Can you work these out from the model? Positions are in its coordinate system, mm. Face numbers are marked on the shaded views. A direction names the side the tool comes from. Coordinates: 2 decimals unless noted, no trailing zeros. Loops run counter-clockwise (first coordinate to the right, second up) from the corner with the lowest first, then second, coordinate; pieces in that order, holes last.
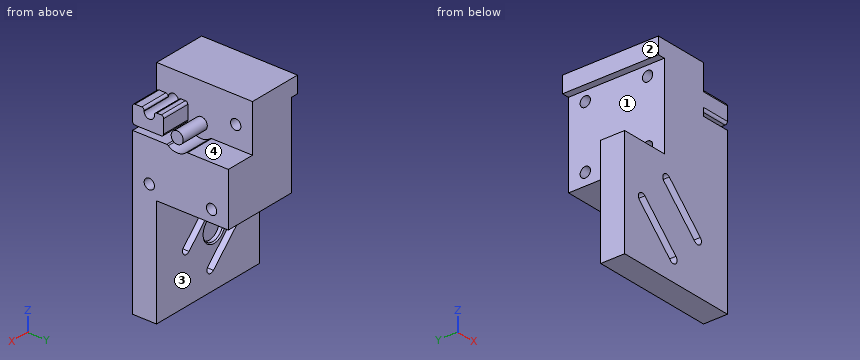
```python
from build123d import *

# Parameters (mm, degrees)
SKETCH3_W             = 13.49028586
SKETCH3_H             = 10
BOSS_EXTRUDE1_DEPTH   = 22
SKETCH3_W_2           = 3
BOSS_EXTRUDE1_2_DEPTH = 22
BOSS_EXTRUDE1_3_DEPTH = 22
SKETCH4_W             = 27.150730292
SKETCH4_H             = 10
BOSS_EXTRUDE2_DEPTH   = 3
SKETCH5_W             = 27.150730292
SKETCH5_H             = 10
BOSS_EXTRUDE3_DEPTH   = 3
SKETCH7_W             = 12.1
SKETCH7_H             = 14.76
BOSS_EXTRUDE4_DEPTH   = 10
BOSS_EXTRUDE5_DEPTH   = 10
SKETCH15_R            = 1.915111108
CUT_EXTRUDE4_DEPTH    = 320.517471197
SKETCH18_W            = 12.1
SKETCH18_H            = 14.76
BOSS_EXTRUDE6_DEPTH   = 30
M4_CLEARANCE_HOLE1_D  = 4.3
CUT_EXTRUDE7_DEPTH    = 5
SKETCH17_R            = 5
CUT_EXTRUDE6_DEPTH    = 2
CHAMFER1_SIZE         = 0.5
SKETCH24_W            = 5
SKETCH24_H            = 40
CUT_EXTRUDE8_DEPTH    = 12.1
SKETCH25_R            = 2.5
BOSS_EXTRUDE10_DEPTH  = 12.1
CUT_EXTRUDE10_START   = -12.1
SKETCH31_R            = 5.628705003
SKETCH31_R_2          = 2.5
CUT_EXTRUDE10_DEPTH   = 12.1
FILLET1_R             = 1


with BuildPart() as part:
    # Sketch3 → Boss-Extrude1 (new body)
    with BuildSketch(Plane(origin=(-188.9, 0, 188.9), x_dir=(0.7071067811865475, 0, 0.7071067811865477), z_dir=(-0.7071067811865477, 0, 0.7071067811865475))):
        with Locations((0, -11.606969024)):
            Rectangle(SKETCH3_W, SKETCH3_H)
    extrude(amount=-BOSS_EXTRUDE1_DEPTH)



with BuildPart() as body_2:
    # Sketch3 → Boss-Extrude1 2 (new body)
    with BuildSketch(Plane(origin=(-188.9, 0, 188.9), x_dir=(0.7071067811865475, 0, 0.7071067811865477), z_dir=(-0.7071067811865477, 0, 0.7071067811865475))):
        with Locations((12.075365146, -11.606969024)):
            Rectangle(SKETCH3_W_2, SKETCH3_H)
    extrude(amount=-BOSS_EXTRUDE1_2_DEPTH)


with BuildPart() as body_3:
    # Sketch3 → Boss-Extrude1 3 (new body)
    with BuildSketch(Plane(origin=(-188.9, 0, 188.9), x_dir=(0.7071067811865475, 0, 0.7071067811865477), z_dir=(-0.7071067811865477, 0, 0.7071067811865475))):
        with Locations((-12.075365146, -11.606969024)):
            Rectangle(SKETCH3_W_2, SKETCH3_H)
    extrude(amount=-BOSS_EXTRUDE1_3_DEPTH)


with BuildPart() as part_1:
    add(part.part)

    add(body_2.part)  # Boss-Extrude2 merges body 2

    add(body_3.part)  # Boss-Extrude2 merges body 3
    # Sketch4 → Boss-Extrude2 (add)
    with BuildSketch(Plane(origin=(-188.9, 0, 188.9), x_dir=(0.7071067811865472, 0, 0.7071067811865479), z_dir=(-0.7071067811865479, 0, 0.7071067811865472))):
        with Locations((0, -11.606969024)):
            Rectangle(SKETCH4_W, SKETCH4_H)
    extrude(amount=BOSS_EXTRUDE2_DEPTH)

    # Sketch5 → Boss-Extrude3 (add)
    with BuildSketch(Plane(origin=(-173.343650814, 0, 173.343650814), x_dir=(-0.7071067811865472, 0, -0.7071067811865479), z_dir=(0.7071067811865479, 0, -0.7071067811865472))):
        with Locations((0, -11.606969024)):
            Rectangle(SKETCH5_W, SKETCH5_H)
    extrude(amount=BOSS_EXTRUDE3_DEPTH)

    # Sketch7 → Boss-Extrude4 (add)
    with BuildSketch(Plane(origin=(0, -6.606969024, 0), x_dir=(1, 0, 0), z_dir=(0, 1, 0))):
        Polygon((-183.9, -239), (-186.9, -239), (-186.9, -245.88), (-147.25, -245.88), (-147.25, -161.623097719), (-180.821563222, -161.623097719), (-161.623097719, -180.821563222), (-181.422087592, -200.620553095), (-200.620553095, -181.422087592), (-200.620553095, -203.8), (-183.9, -203.8), align=None)
        with Locations((-158.3, -233.5)):
            Rectangle(SKETCH7_W, SKETCH7_H, mode=Mode.SUBTRACT)
    extrude(amount=-BOSS_EXTRUDE4_DEPTH)

    # Sketch13 → Boss-Extrude5 (add)
    with BuildSketch(Plane(origin=(0, -6.606969024, 0), x_dir=(1, 0, 0), z_dir=(0, 1, 0))):
        Polygon((-203.8, -203.8), (-200.620553095, -203.8), (-200.620553095, -181.422087592), (-180.821563222, -161.623097719), (-147.25, -161.623097719), (-147.25, -158.443650814), (-203.8, -158.443650814), align=None)
    extrude(amount=-BOSS_EXTRUDE5_DEPTH)

    # Sketch15 → Cut-Extrude4 (cut, through all)
    with BuildSketch(Plane(origin=(0, -6.606969024, 0), x_dir=(1, 0, 0), z_dir=(0, 1, 0))):
        with Locations((-179.467375171, -167.219926457)):
            Circle(SKETCH15_R)
        with Locations((-167.219926457, -179.467375171)):
            Circle(SKETCH15_R)
        with Locations((-195.023724357, -182.776275643)):
            Circle(SKETCH15_R)
        with Locations((-182.776275643, -195.023724357)):
            Circle(SKETCH15_R)
    extrude(amount=-CUT_EXTRUDE4_DEPTH, mode=Mode.SUBTRACT)

    # Sketch18 → Boss-Extrude6 (add)
    with BuildSketch(Plane(origin=(0, -6.606969024, 0), x_dir=(1, 0, 0), z_dir=(0, 1, 0))):
        Polygon((-183.9, -203.8), (-147.25, -203.8), (-147.25, -245.88), (-186.9, -245.88), (-186.9, -239), (-183.9, -239), align=None)
        with Locations((-158.3, -233.5)):
            Rectangle(SKETCH18_W, SKETCH18_H, mode=Mode.SUBTRACT)
    extrude(amount=BOSS_EXTRUDE6_DEPTH)

    # M4 Clearance Hole1 (through all)
    with Locations(Plane(origin=(-147.25, 0, 0), x_dir=(0, 0, -1), z_dir=(1, 0, 0))):
        with Locations((-234.9, 16.393030976), (-208.9, -9.606969024), (-234.9, -9.606969024), (-208.9, 16.393030976)):
            Hole(M4_CLEARANCE_HOLE1_D / 2)

    # Sketch22 → Cut-Extrude7 (cut)
    with BuildSketch(Plane(origin=(-147.25, 0, 0), x_dir=(0, 0, -1), z_dir=(1, 0, 0))):
        Polygon((-245.88, 23.393030976), (-245.88, -16.606969024), (-158.443650814, -16.606969024), (-158.443650814, -6.606969024), (-203.8, -6.606969024), (-203.8, 23.393030976), align=None)
    extrude(amount=-CUT_EXTRUDE7_DEPTH, mode=Mode.SUBTRACT)

    # Sketch17 → Cut-Extrude6 (cut)
    with BuildSketch(Plane(origin=(0, -6.606969024, 0), x_dir=(1, 0, 0), z_dir=(0, 1, 0))):
        with Locations(Location((-181.121825407, -181.121825407, 0), (0, 0, 270))):
            Circle(SKETCH17_R)
    extrude(amount=-CUT_EXTRUDE6_DEPTH, mode=Mode.SUBTRACT)

    # Chamfer1
    chamfer1_edges = [part_1.edges().sort_by_distance(p)[0] for p in [
        (-181.121825407, -6.606969024, 176.121825407),
    ]]
    chamfer(chamfer1_edges, length=CHAMFER1_SIZE)

    # Sketch24 → Cut-Extrude8 (cut)
    with BuildSketch(Plane(origin=(-152.25, 0, 0), x_dir=(0, 0, -1), z_dir=(1, 0, 0))):
        with Locations((-243.38, 3.393030976)):
            Rectangle(SKETCH24_W, SKETCH24_H)
    extrude(amount=-CUT_EXTRUDE8_DEPTH, mode=Mode.SUBTRACT)

    # Sketch25 → Boss-Extrude10 (add)
    with BuildSketch(Plane(origin=(-164.35, 0, 0), x_dir=(0, 0, -1), z_dir=(1, 0, 0))):
        with Locations(Location((-230.14, 2.021735979, 0), (0, 0, 270))):
            Circle(SKETCH25_R)
        with BuildLine():
            Line((-228.41, -3.606969024), (-236.12, -3.606969024))
            Line((-236.12, -3.606969024), (-236.12, -7.456969024))
            Line((-236.12, -7.456969024), (-234.9, -7.456969024))
            ThreePointArc((-234.9, -7.456969024), (-232.75, -9.606969024), (-234.9, -11.756969024))
            Line((-234.9, -11.756969024), (-236.12, -11.756969024))
            Line((-236.12, -11.756969024), (-236.12, -16.606969024))
            Line((-236.12, -16.606969024), (-228.41, -16.606969024))
            Line((-228.41, -16.606969024), (-228.41, -3.606969024))
        make_face()
    extrude(amount=BOSS_EXTRUDE10_DEPTH)

    # Sketch31 → Cut-Extrude10 (cut)
    with BuildSketch(Plane(origin=(-152.25, 0, 0), x_dir=(0, 0, -1), z_dir=(1, 0, 0)).offset(CUT_EXTRUDE10_START)):
        with Locations((-230.14, 2.021735979)):
            Circle(SKETCH31_R)
        with Locations(Location((-230.14, 2.021735979, 0), (0, 0, 270))):
            Circle(SKETCH31_R_2, mode=Mode.SUBTRACT)
    extrude(amount=CUT_EXTRUDE10_DEPTH, mode=Mode.SUBTRACT)

    # Fillet1
    fillet1_edges = [part_1.edges().sort_by_distance(p)[0] for p in [
        (-158.3, -16.606969024, 228.41),
        (-158.3, -3.606969024, 228.41),
        (-158.3, -3.606969024, 236.12),
        (-158.3, -7.456969024, 236.12),
        (-158.3, -11.756969024, 236.12),
        (-158.3, -16.606969024, 236.12),
        (-158.3, 5.961522777, 226.12),
        (-158.3, -1.918050819, 226.12),
    ]]
    fillet(fillet1_edges, radius=FILLET1_R)


solid = part_1.part
```
(1) I want a section at D-D on z = 195.5. Write out the boundary of the cut face in (x, y), then the cut area to 3 significant figures.
Check values:
outline: (-203.8, -16.61) - (-184.63, -16.61) - (-184.63, -6.61) - (-203.8, -6.61) - close; (-180.54, -16.61) - (-152.25, -16.61) - (-152.25, -6.61) - (-180.54, -6.61) - close
area: 475 mm2
(2) If I drill on probe 1 along Z at (x, y) = (-183.5, 14.5); probe 2 along Z at (x, y) = (-180, 18); probe 3 along X at (y, z) = (-11.5, 184), over which ranges is the centre line in solid material (lowest first)?
Check values:
probe 1: z = 203.8 to 207.88, 209.92 to 233.88, 235.92 to 245.88
probe 2: z = 203.8 to 207.47, 210.33 to 233.47, 236.33 to 245.88
probe 3: x = -203.8 to -196.5, -193.54 to -174.46, -169.04 to -152.25
(3) I'm going to push flat-ended pins straight in: pin 1 (2.5 mm diameter, centred on y = -9.61, z = 234.9, fed in from -X); pin 2 (15 mm diameter, centred on x = -167.5, y = 15, fed in from -Z); pin 3 (3 mm diameter, centred on x = -183.5, z = 179, fed in from +Y); pin 4 (2.5 mm diameter, centred on x = -156.5, y = -13.5, fed in from +Z). Where does each tip first touch, or does it pass through?
Check values:
pin 1: passes through
pin 2: stops at z = 203.8
pin 3: stops at y = -8.61
pin 4: stops at z = 236.12
(4) I want a section at A-A on z = 208.9. Write out the boundary of the cut face in (x, y), then the cut area to 3 significant figures.
Check values:
outline: (-183.9, -16.61) - (-152.25, -16.61) - (-152.25, -11.76) - (-183.9, -11.76) - close; (-183.9, -7.46) - (-152.25, -7.46) - (-152.25, 14.24) - (-183.9, 14.24) - close; (-183.9, 18.54) - (-152.25, 18.54) - (-152.25, 23.39) - (-183.9, 23.39) - close
area: 994 mm2
(5) Which directions (+Z, -Z, +X, -X, +Y, -Y) give clear straight access to the entire face, cutting with the end or side of a thin tool? Please do the marked faces 1, 2, 3 and 4.
Check values:
face 1: -X, +Y, -Y
face 2: +Z, -X, +Y, -Y
face 3: -Z, +X, -X, +Y
face 4: +Z, +X, +Y, -Y
(6) I want a section at C-C on y = 11. Write out the boundary of the cut face in (x, z), then the cut area to 3 significant figures.
Check values:
outline: (-186.9, 239) - (-183.9, 239) - (-183.9, 203.8) - (-152.25, 203.8) - (-152.25, 226.12) - (-164.35, 226.12) - (-164.35, 245.88) - (-186.9, 245.88) - close
area: 1,110 mm2
(7) I want a section at B-B on x = -174. Write out the boundary of the cut face in (y, z).
Check values:
outline: (-16.61, 158.44) - (-6.61, 158.44) - (-6.61, 183.54) - (-16.61, 183.54) - close; (-16.61, 188.96) - (-6.61, 188.96) - (-6.61, 203.8) - (23.39, 203.8) - (23.39, 245.88) - (-16.61, 245.88) - close; hole circle Ø4.3 at (-9.61, 208.9); hole circle Ø4.3 at (-9.61, 234.9); hole circle Ø4.3 at (16.39, 208.9); hole circle Ø4.3 at (16.39, 234.9)
